```python
from build123d import *

# Parameters (mm, degrees)
F0_W      = 54.864
F0_H      = 34.29
F1_DEPTH  = 28.575
F2_T      = -3.175
F3_W      = 5.334
F3_H      = 7.112
F4_DEPTH  = 3.81
F6_DEPTH  = 54.864
F8_D      = 2.794
F8_DEPTH  = 10.16
F9_W      = 12.7
F9_H      = 7.62
F10_DEPTH = 3.175


with BuildPart() as f1:
    # F0 (on Top) → F1 (new body)
    with BuildSketch(Plane.XY):
        with Locations((1.706375, 0)):
            Rectangle(F0_W, F0_H)
    extrude(amount=F1_DEPTH)

    # F2
    f2_openings = [f1.faces().sort_by_distance(p)[0] for p in [
        (1.706375, 0, 28.575),
    ]]
    offset(amount=F2_T, openings=f2_openings)

    # F3 (on face) → F4 (join)
    with BuildSketch(Plane.XY.offset(3.175)):
        with Locations((-19.883625, 10.414)):
            Rectangle(F3_W, F3_H)
        with Locations((-19.883625, -10.414)):
            Rectangle(F3_W, F3_H)
        with Locations((23.296375, -10.414)):
            Rectangle(F3_W, F3_H)
        with Locations((23.296375, 10.414)):
            Rectangle(F3_W, F3_H)
    extrude(amount=F4_DEPTH)

    # F5 (on face) → F6 (join)
    with BuildSketch(Plane.YZ.offset(29.138375)):
        Polygon((17.145, -6.35), (17.145, 0), (-17.145, 0), (-17.145, -6.35), (-10.795, -6.35), (-13.97, -3.175), (-10.795, -3.175), (13.97, -3.175), (10.795, -6.35), align=None)
    extrude(amount=-F6_DEPTH)

    # F8
    with Locations(Plane.XY.offset(6.985)):
        with Locations((-20.340825, 11.7602), (23.677375, 11.684), (23.677375, -11.684), (-20.340825, -11.7602)):
            Hole(F8_D / 2, depth=F8_DEPTH)

    # F9 (on face) → F10 (cut)
    with BuildSketch(Plane(origin=(-25.725625, 0, 0), x_dir=(0, -1, 0), z_dir=(-1, 0, 0))):
        with Locations((0, 5.461)):
            Rectangle(F9_W, F9_H)
    extrude(amount=-F10_DEPTH, mode=Mode.SUBTRACT)


solid = f1.part
```
For this review, take the finished solid that the model builds, in its own axes (mm). A direction names the side the tool comes from. Coordinates: 2 decimals unless noted, no trailing zeros. Loops run counter-clockwise (first coordinate to the right, second up) from the corner with the lowest first, then second, coordinate; pieces in that order, holes last. Notation, with made-up numbers: (1, -2.5) - (54, -2.5) arc R26 cw to (54, 27.5) - close; hole circle Ø8 at (-15.75, 18). An arc over 180 degrees is marked (long way). Use one line per item in the form item = value. Start each with the question number.
1) Take a section at D-D (y = 8). State the section outline as (x, z) points (3 decimals).
2) For faces 1 (the face through (2.09, -12.36, -4.785)), 2 (the face through (-24, -6.35, 5)), 3 (the face through (23, 10, 6.985)), list the 3-axis set-ups (+Z, -Z, +X, -X, +Y, -Y) from which the entire face can be reached by the end or side of a thin tool; tool diameter is ignored.
3) Take a section at C-C (x = 0). State the section outline as (y, z) points (3 decimals), plus the area to 3 significant figures.
4) Take a section at A-A (y = -5). State the section outline as (x, z) points (3 decimals).
5) Take a section at B-B (z = 22). State the section outline as (x, y) points (3 decimals).
6) For pin 1 (1 mm diameter, centred on x = -19.5, y = -8, fed in from -Z) (3 decimals); pin 2 (14 mm diameter, centred on x = 12.5, y = -0.5, fed in from +Z) (3 decimals); pin 3 (0.5 mm diameter, centred on y = -3, z = 2.5, fed in from -X), all flat-tipped, find the tip position at first contact; note any pin that passes through.
7) Draft analysis for pull direction Y (two halves, no side actions). For faces 4 (the face through (2.09, 12.405, -4.74)), 5 (the face through (2, 17.145, 11)), 6 (the face through (0, 15, 28.575)), state which applies: released by +Y, released by -Y, zero draft, split by the parting line, or undercut.
8) To check wall thickness, follow probe 1 along X at (y, z) = (13.5, 6.5); probe 2 along Y at (x, z) = (10.5, 24) (3 decimals); probe 3 along X at (y, z) = (-4.5, 23). State the ranges of each line that lie inside material, in increasing order. Write a range as from..to.
From the geometry:
q1.outline = (-25.726, -3.175) - (29.138, -3.175) - (29.138, 28.575) - (25.963, 28.575) - (25.963, 6.985) - (20.629, 6.985) - (20.629, 3.175) - (-17.217, 3.175) - (-17.217, 6.985) - (-22.551, 6.985) - (-22.551, 28.575) - (-25.726, 28.575) - close
q2.face_1 = +X, -X
q2.face_2 = -X
q2.face_3 = +Z
q3.outline = (-17.145, -6.35) - (-10.795, -6.35) - (-13.97, -3.175) - (13.97, -3.175) - (10.795, -6.35) - (17.145, -6.35) - (17.145, 28.575) - (13.97, 28.575) - (13.97, 3.175) - (-13.97, 3.175) - (-13.97, 28.575) - (-17.145, 28.575) - close
q3.area = 409 mm2
q4.outline = (-25.726, -3.175) - (29.138, -3.175) - (29.138, 28.575) - (25.963, 28.575) - (25.963, 3.175) - (-22.551, 3.175) - (-22.551, 1.651) - (-25.726, 1.651) - close; (-25.726, 9.271) - (-22.551, 9.271) - (-22.551, 28.575) - (-25.726, 28.575) - close
q5.outline = (-25.726, -17.145) - (29.138, -17.145) - (29.138, 17.145) - (-25.726, 17.145) - close; hole (-22.551, -13.97) - (25.963, -13.97) - (25.963, 13.97) - (-22.551, 13.97) - close
q6.pin_1 = -3.175
q6.pin_2 = 3.175
q6.pin_3 = -22.55
q7.face_4 = undercut
q7.face_5 = released by +Y
q7.face_6 = zero draft
q8.probe_1 = -25.73..-17.22, 20.63..29.14
q8.probe_2 = -17.145..-13.97, 13.97..17.145
q8.probe_3 = -25.73..-22.55, 25.96..29.14
